Autodesk Inventor part; units mm, degrees
ref_plane "YZ Plane" through (0, 0, 0) normal (1, 0, 0) x (0, 1, 0)
ref_plane "XZ Plane" through (0, 0, 0) normal (0, 1, 0) x (-1, 0, 0)
ref_plane "XY Plane" through (0, 0, 0) normal (0, 0, 1) x (1, 0, 0)
sketch "草图1" plane through (0, 0, 0) normal (0, 0, 1) x (1, 0, 0)
  line L0 (-100, 100) -> (100, 100)
  line L1 (100, 100) -> (100, -100)
  line L2 (100, -100) -> (-100, -100)
  line L3 (-100, -100) -> (-100, 100)
  line L4 (-100, 100) -> (100, -100) construction
  line L5 (100, 100) -> (-100, -100) construction
  point P0 (0, 0)
  dimension "d0" = 200
  dimension "d1" = 200
extrude "拉伸1" add sketch "草图1" along normal blind 250
sketch "草图3" plane through (0, 0, 250) normal (0, 0, 1) x (1, 0, 0)
  line L0 (-90, 90) -> (90, 90)
  line L1 (90, 90) -> (90, -90)
  line L2 (90, -90) -> (-90, -90)
  line L3 (-90, -90) -> (-90, 90)
  line L4 (-90, 90) -> (90, -90) construction
  line L5 (90, 90) -> (-90, -90) construction
  point P0 (0, 0)
  dimension "d6" = 180
  dimension "d7" = 180
extrude "拉伸2" add sketch "草图3" along normal blind 3
chamfer "倒角1" distance 40 angle 45 4 edges at (100, 100, 125) (-100, -100, 125) (100, -100, 125) (-100, 100, 125)
sketch "草图4" plane through (0, 0, 253) normal (0, 0, 1) x (1, 0, 0)
  line L0 (-100, 100) -> (100, 100)
  line L1 (100, 100) -> (100, -100)
  line L2 (100, -100) -> (-100, -100)
  line L3 (-100, -100) -> (-100, 100)
  line L4 (-100, 100) -> (100, -100) construction
  line L5 (100, 100) -> (-100, -100) construction
  point P0 (0, 0)
  dimension "d10" = 200
  dimension "d11" = 200
extrude "拉伸3" add sketch "草图4" along normal blind 20
sketch "草图5" plane through (0, 0, 273) normal (0, 0, 1) x (1, 0, 0)
  circle A0 centre (0, 0) radius 50
  dimension "d17" = 100
extrude "拉伸4" add sketch "草图5" along normal blind 20
fillet "圆角1" radius 10 1 edges at (-50, 0, 293)
sketch "草图6" plane through (0, 0, 273) normal (0, 0, 1) x (1, 0, 0)
  circle A0 centre (0, 0) radius 65
  dimension "d21" = 130
extrude "拉伸5" add sketch "草图6" along normal blind 1
sketch "草图7" plane through (0, 0, 293) normal (0, 0, 1) x (1, 0, 0)
  circle A0 centre (0, 0) radius 30
  dimension "d24" = 60
extrude "拉伸6" cut sketch "草图7" against normal blind 15
sketch "草图8" plane through (0, 0, 278) normal (0, 0, 1) x (1, 0, 0)
  circle A0 centre (0, 0) radius 17.5
  dimension "d27" = 35
extrude "拉伸7" add sketch "草图8" along normal blind 10
sketch "草图9" plane through (0, 0, 288) normal (0, 0, 1) x (1, 0, 0)
  circle A0 centre (0, 0) radius 15
  dimension "d30" = 30
extrude "拉伸8" add sketch "草图9" along normal blind 80
sketch "草图10" plane through (0, 0, 273) normal (0, 0, 1) x (1, 0, 0)
  point P0 (0, 0)
  point P1 (-60, 60)
  point P2 (60, 60)
  point P3 (60, -60)
  point P4 (-60, -60)
  dimension "d33" = 60
  dimension "d34" = 60
  dimension "d37" = 360
hole "孔1" at (-60, 60, 273) at (60, 60, 273) at (60, -60, 273) at (-60, -60, 273) direction (0, 0, -1) diameter 20.752 depth 61.1 tip angle 118
chamfer "倒角2" distance 20 angle 45 4 edges at (-100, -100, 263) (100, -100, 263) (100, 100, 263) (-100, 100, 263)
scale "缩放比例1" factors (0.4, 0.4, 0.4) then translate (0, 0, 0) bodies 1
properties part number "电机"
Input: part model. Units: mm. Frame: model coordinates. A direction names the side the tool comes from. Coordinates: 2 decimals unless noted, no trailing zeros. Loops run counter-clockwise (first coordinate to the right, second up) from the corner with the lowest first, then second, coordinate; pieces in that order, holes last.
Q1. Mould query, pull axis Y, two halves, no side actions, for faces 1 (the flat face through (-36, 36, 105)), 2 (the flat face through (5.2, -5.2, 111.2)), 3 (the cylindrical face through (-20.633, 15.821, 109.397)). Classes: +Y half, -Y half, draft (parallel to the pull), parting line (faces both ways), or undercut.
Results are:
face 1: +Y half
face 2: undercut
face 3: parting line
Q2. Section A-A, the plane z = 87.5. Return the cut outline in (x, y).
Results are:
outline: (-40, -24) - (-24, -40) - (24, -40) - (40, -24) - (40, 24) - (24, 40) - (-24, 40) - (-40, 24) - close; hole circle Ø8.3 at (-24, -24); hole circle Ø8.3 at (-24, 24); hole circle Ø8.3 at (24, -24); hole circle Ø8.3 at (24, 24)
Q3. Contact query for flat-ended pins moving along their axis: pin 1 (0.6 mm diameter, centred on x = 13.5, z = 100.5, fed in from -Y); pin 2 (13.5 mm diameter, centred on x = -24, y = -24, fed in from +Z); pin 3 (6 mm diameter, centred on x = 28.5, z = 66, fed in from -Y). Output: stop coordinate, or through.
Results are:
pin 1: stops at y = -36
pin 2: stops at z = 109.2
pin 3: stops at y = -38.5
Q4. Line query: line 1 along Y through (x, z) = (24, 97.75); line 2 along Y through (x, z) = (0, 113.15). Output: solid intervals per line, ascending.
Results are:
line 1: y = -40 to -28.15, -19.85 to 19.85, 28.15 to 40
line 2: y = -20 to -12, -7 to 7, 12 to 20
Q5. Set-up query: faces 4 (the cylindrical face through (-11.99, 0.53, 114.24)), 5 (the flat face through (-38, 0, 100)), 6 (the flat face through (32, -32, 50)), 7 (the flat face through (-32, 32, 50)). Return all of +Z, -Z, +X, -X, +Y, -Y with unobstructed straight access to the full face (end or side cutting, diameter ignored); none if empty.
Results are:
face 4: +Z
face 5: -X, +Y, -Y
face 6: -Z, +X, -Y
face 7: -Z, -X, +Y
